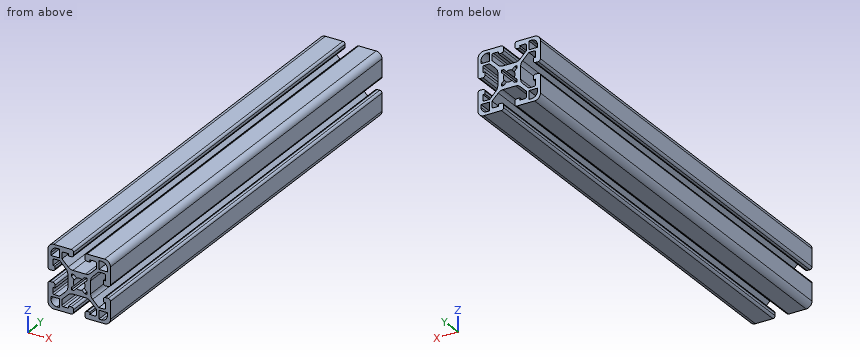
from build123d import *

# Parameters (mm, degrees)
SKETCH1_W           = 4.9403
SKETCH1_H           = 4.9403
BOSS_EXTRUDE6_DEPTH = 254
FILLET1_R           = 3.4125154
FILLET2_R           = 0.762
FILLET3_R           = 1.27
FILLET4_R           = 3.81


with BuildPart() as part:
    # Sketch1 → Boss-Extrude6 (new body)
    with BuildSketch(Plane(origin=(0, 0, 0), x_dir=(1, 0, 0), z_dir=(0, 1, 0))):
        Polygon((-7.366, -7.366), (7.366, -7.366), (7.366, -3.302), (4.510882512, -3.302), (4.572, -4.572), (0.7239, -4.572), (0.7239, -0.64109893), (5.404132197, 4.039133267), (15.856734336, 4.039133267), (20.536966533, -0.64109893), (20.536966533, -4.572), (16.688866533, -4.572), (16.749984021, -3.302), (13.894866533, -3.302), (13.894866533, -7.366), (28.626866533, -7.366), (28.626866533, 7.366), (24.562866533, 7.366), (24.562866533, 4.510882512), (25.832866533, 4.572), (25.832866533, 0.7239), (21.901965464, 0.7239), (17.221733267, 5.404132197), (17.221733267, 15.856734336), (21.901965464, 20.536966533), (25.832866533, 20.536966533), (25.832866533, 16.688866533), (24.562866533, 16.749984021), (24.562866533, 13.894866533), (28.626866533, 13.894866533), (28.626866533, 28.626866533), (13.894866533, 28.626866533), (13.894866533, 24.562866533), (16.749984021, 24.562866533), (16.688866533, 25.832866533), (20.536966533, 25.832866533), (20.536966533, 21.901965464), (15.856734336, 17.221733267), (5.404132197, 17.221733267), (0.7239, 21.901965464), (0.7239, 25.832866533), (4.572, 25.832866533), (4.510882512, 24.562866533), (7.366, 24.562866533), (7.366, 28.626866533), (-7.366, 28.626866533), (-7.366, 13.894866533), (-3.302, 13.894866533), (-3.302, 16.749984021), (-4.572, 16.688866533), (-4.572, 20.536966533), (-0.64109893, 20.536966533), (4.039133267, 15.856734336), (4.039133267, 5.404132197), (-0.64109893, 0.7239), (-4.572, 0.7239), (-4.572, 4.572), (-3.302, 4.510882512), (-3.302, 7.366), (-7.366, 7.366), align=None)
        with Locations((-3.19405, -3.19405)):
            Rectangle(SKETCH1_W, SKETCH1_H, mode=Mode.SUBTRACT)
        with Locations((-3.19405, 24.454916533)):
            Rectangle(SKETCH1_W, SKETCH1_H, mode=Mode.SUBTRACT)
        with Locations((24.454916533, 24.454916533)):
            Rectangle(SKETCH1_W, SKETCH1_H, mode=Mode.SUBTRACT)
        with Locations((24.454916533, -3.19405)):
            Rectangle(SKETCH1_W, SKETCH1_H, mode=Mode.SUBTRACT)
        with BuildLine():
            Line((7.696270003, 12.1995976), (6.157493267, 13.738374336))
            Line((6.157493267, 13.738374336), (6.157493267, 15.103373267))
            Line((6.157493267, 15.103373267), (7.522492197, 15.103373267))
            Line((7.522492197, 15.103373267), (9.061268934, 13.56459653))
            ThreePointArc((9.061268934, 13.56459653), (10.630433267, 13.957833267), (12.1995976, 13.56459653))
            Line((12.1995976, 13.56459653), (13.738374336, 15.103373267))
            Line((13.738374336, 15.103373267), (15.103373267, 15.103373267))
            Line((15.103373267, 15.103373267), (15.103373267, 13.738374336))
            Line((15.103373267, 13.738374336), (13.56459653, 12.1995976))
            ThreePointArc((13.56459653, 12.1995976), (13.957833267, 10.630433267), (13.56459653, 9.061268934))
            Line((13.56459653, 9.061268934), (15.103373267, 7.522492197))
            Line((15.103373267, 7.522492197), (15.103373267, 6.157493267))
            Line((15.103373267, 6.157493267), (13.738374336, 6.157493267))
            Line((13.738374336, 6.157493267), (12.1995976, 7.696270003))
            ThreePointArc((12.1995976, 7.696270003), (10.630433267, 7.303033267), (9.061268934, 7.696270003))
            Line((9.061268934, 7.696270003), (7.522492197, 6.157493267))
            Line((7.522492197, 6.157493267), (6.157493267, 6.157493267))
            Line((6.157493267, 6.157493267), (6.157493267, 7.522492197))
            Line((6.157493267, 7.522492197), (7.696270003, 9.061268934))
            ThreePointArc((7.696270003, 9.061268934), (7.303033267, 10.630433267), (7.696270003, 12.1995976))
        make_face(mode=Mode.SUBTRACT)
    extrude(amount=BOSS_EXTRUDE6_DEPTH)

    # Fillet1
    fillet1_edges = [part.edges().sort_by_distance(p)[0] for p in [
        (-7.366, 127, 7.366),
        (-7.366, 127, -28.626866533),
        (28.626866533, 127, -28.626866533),
        (28.626866533, 127, 7.366),
        (26.925066533, 127, 5.6642),
        (26.925066533, 127, -26.925066533),
        (-5.6642, 127, -26.925066533),
        (-5.6642, 127, 5.6642),
    ]]
    fillet(fillet1_edges, radius=FILLET1_R)

    # Fillet2
    fillet2_edges = [part.edges().sort_by_distance(p)[0] for p in [
        (0.7239, 127, 4.572),
        (-4.572, 127, -0.7239),
        (-4.572, 127, -20.536966533),
        (0.7239, 127, -25.832866533),
        (20.536966533, 127, -25.832866533),
        (25.832866533, 127, -20.536966533),
        (25.832866533, 127, -0.7239),
        (20.536966533, 127, 4.572),
    ]]
    fillet(fillet2_edges, radius=FILLET2_R)

    # Fillet3
    fillet3_edges = [part.edges().sort_by_distance(p)[0] for p in [
        (7.366, 127, 3.302),
        (7.366, 127, 7.366),
        (-7.366, 127, -7.366),
        (-3.302, 127, -7.366),
        (-3.302, 127, -13.894866533),
        (-7.366, 127, -13.894866533),
        (7.366, 127, -28.626866533),
        (7.366, 127, -24.562866533),
        (13.894866533, 127, -24.562866533),
        (13.894866533, 127, -28.626866533),
        (28.626866533, 127, -13.894866533),
        (24.562866533, 127, -13.894866533),
        (24.562866533, 127, -7.366),
        (28.626866533, 127, -7.366),
        (13.894866533, 127, 7.366),
        (13.894866533, 127, 3.302),
    ]]
    fillet(fillet3_edges, radius=FILLET3_R)

    # Fillet4
    fillet4_edges = [part.edges().sort_by_distance(p)[0] for p in [
        (4.039133267, 127, -5.404132197),
        (4.039133267, 127, -15.856734336),
        (5.404132197, 127, -17.221733267),
        (15.856734336, 127, -17.221733267),
        (17.221733267, 127, -15.856734336),
        (17.221733267, 127, -5.404132197),
        (15.856734336, 127, -4.039133267),
        (5.404132197, 127, -4.039133267),
    ]]
    fillet(fillet4_edges, radius=FILLET4_R)


solid = part.part
Geometry: final body of the model. Coordinates: model frame, mm. Coordinates: 2 decimals unless noted, no trailing zeros.
(1) First-contact query: pin 1 (1.1 mm diameter, centred on y = 155, z = -7, fed in from -X); pin 2 (0.8 mm diameter, centred on x = -5.5, y = 175, fed in from -Z); pin 3 (2 mm diameter, centred on x = 0, z = -5, fed in from +Y); pin 4 (1.1 mm diameter, centred on x = 7, y = 134.5, fed in from +Z). Flat tips, straight axial feed; report the tip coordinate or a pass-through.
(2) Material intervals for probe 1 along X at (y, z) = (172.5, 2.5); probe 2 along Z at (x, y) = (17, 34.5) (3 decimals); probe 3 along Z at (x, y) = (18, 103) (3 decimals), sorted ascending.
(3) Section query A-A (y = 222.5). State how many separate pieces and enclosed holes the cut face has, plus the area to 3 significant figures.
Solution:
1. pin 1: stops at x = -7.32
1. pin 2: stops at z = -28.43
1. pin 3: passes through
1. pin 4: stops at z = 7.32
2. probe 1: x = -7.37 to -5.66, -0.72 to 0.72, 20.54 to 21.98, 26.92 to 28.63
2. probe 2: z = -28.627 to -25.833, -18.365 to -2.896, 4.572 to 7.366
2. probe 3: z = -28.627 to -25.833, -19.365 to -16.586, -4.675 to -1.896, 4.572 to 7.366
3. separate pieces: 1
3. enclosed holes: 5
3. area: 502 mm2
